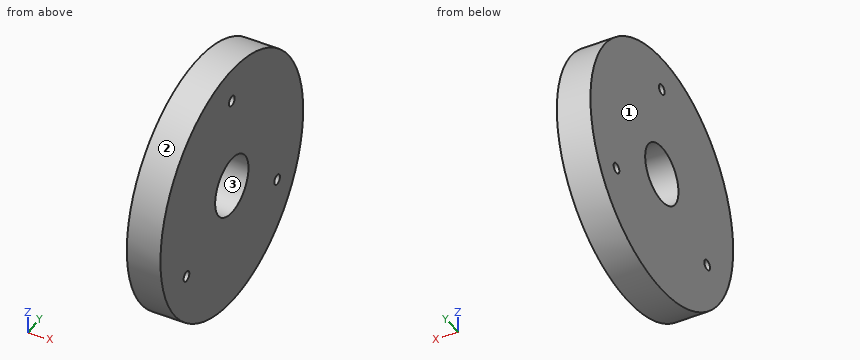
from build123d import *

# Parameters (mm, degrees)
F0_W     = 20
F0_H     = 75
F2_R     = 17.5
F2_R_2   = 3
F3_DEPTH = 20


with BuildPart() as f1:
    # F0 (on Front) → F1 (revolve)
    with BuildSketch(Plane.XZ):
        with Locations((10, -37.5)):
            Rectangle(F0_W, F0_H)
    revolve(axis=Axis((10, 0, 0), (1, 0, 0)))

    # F2 (on Right) → F3 (cut, through all)
    with BuildSketch(Plane.YZ):
        Circle(F2_R)
        with Locations((0, 55)):
            Circle(F2_R_2)
        with Locations((-47.631397, -27.5)):
            Circle(F2_R_2)
        with Locations((47.631397, -27.5)):
            Circle(F2_R_2)
    extrude(amount=F3_DEPTH, mode=Mode.SUBTRACT)


solid = f1.part
Input: part model. Units: mm. Frame: model coordinates. Face numbers are marked on the shaded views. Coordinates: 2 decimals unless noted, no trailing zeros. Order: outer loops, then holes, each group sorted by start corner. A loop starts at its lowest first (then second) coordinate and runs counter-clockwise, first axis right, second up. Notation, with made-up numbers: M 10,85.25 L 49,85.25 A12 ccw 49,102.25 Z; hole C 24.5,-40 d7. An arc over 180 degrees is marked long. Write item = value, one per line. Start each with the question number.
(1) Section C-C on x = 13. Output: boundary loops of the cut face in (y, z).
(2) Section D-D on z = -27.5. Output: boundary loops of the cut face in (x, y), and give its area (3 significant figures).
(3) Pull-direction query (Z, two-part tool) for the marked faces 1, 2 and 3; classes: released by +Z, released by -Z, zero draft, split by the parting line, or undercut.
(4) Line query: line 1 along Z through (x, y) = (18.5, 0.5); line 2 along Y through (x, z) = (8.75, 8); line 3 along Y through (x, z) = (13.25, -13.5) (3 decimals). Output: solid intervals per line, ascending. Write a range as [from, to].
(5) First-contact query: P1, Ø3, axis at y = -50, z = 44, coming from the -X side; P2, Ø4, axis at x = 12.5, y = 51, coming from the +Z side; P3, Ø3, axis at x = 3.5, y = 18.5, coming from the -Z side; P4, Ø2, axis at x = 18, y = 25, coming from the -Z side. Flat tips, straight axial feed; report the tip coordinate or a pass-through.
(6) Section B-B on z = 55. Output: boundary loops of the cut face in (x, y), and give its area (3 significant figures).
(7) Section A-A on y = 0. Output: boundary loops of the cut face in (x, z), and give its area (3 significant figures).
Result set:
q1.outline = C 0,0 d150; hole C -47.63,-27.5 d6; hole C 0,0 d35; hole C 0,55 d6; hole C 47.63,-27.5 d6
q2.outline = M 0,-69.78 L 20,-69.78 L 20,-50.63 L 0,-50.63 Z; M 0,-44.63 L 20,-44.63 L 20,44.63 L 0,44.63 Z; M 0,50.63 L 20,50.63 L 20,69.78 L 0,69.78 Z
q2.area = 2,550 mm²
q3.face_1 = zero draft
q3.face_2 = split by the parting line
q3.face_3 = undercut
q4.line_1 = [-75, -17.49], [17.49, 52.04], [57.96, 75]
q4.line_2 = [-74.57, -15.56], [15.56, 74.57]
q4.line_3 = [-73.775, -11.136], [11.136, 73.775]
q5.P1 = 0
q5.P2 = 56.78
q5.P3 = -73.05
q5.P4 = -71.06
q6.outline = M 0,-50.99 L 20,-50.99 L 20,-3 L 0,-3 Z; M 0,3 L 20,3 L 20,50.99 L 0,50.99 Z
q6.area = 1,920 mm²
q7.outline = M 0,-75 L 20,-75 L 20,-17.5 L 0,-17.5 Z; M 0,17.5 L 20,17.5 L 20,52 L 0,52 Z; M 0,58 L 20,58 L 20,75 L 0,75 Z
q7.area = 2,180 mm²
